Could you check a few things on this model? Use its own coordinates, in mm. A direction names the side the tool comes from. Give positions to 0.01 mm unless a question says otherwise; leave off trailing zeros. Order: outer loops, then holes, each group sorted by start corner. A loop starts at its lowest first (then second) coordinate and runs counter-clockwise, first axis right, second up. Notation, with made-up numbers: M 61,72.25 L 106,72.25 A23 cw 106,107.25 Z; hole C 49,5.25 d3. An arc over 180 degrees is marked long. Return JSON: item names as keys, results as strings. Group by question number.
```python
from build123d import *

# Parameters (mm, degrees)
SKETCH1_W           = 300
SKETCH1_H           = 152
BOSS_EXTRUDE1_DEPTH = 62
CUT_EXTRUDE2_DEPTH  = 342.976607387
SKETCH7_R           = 45
SKETCH7_R_2         = 46.06
SKETCH7_R_3         = 22
CUT_EXTRUDE4_DEPTH  = 339.496676498
CUT_EXTRUDE6_DEPTH  = 339.496676498
CUT_EXTRUDE9_DEPTH  = 339.496676498
SHELL2_DEPTH        = 57
CUT_EXTRUDE10_DEPTH = 55


# Read off the part's stored shape, not the designer's step: Shell2
with BuildPart() as part:
    # Sketch1 → Boss-Extrude1 (new body)
    with BuildSketch(Plane.XY):
        with Locations((150, -76)):
            Rectangle(SKETCH1_W, SKETCH1_H)
    extrude(amount=BOSS_EXTRUDE1_DEPTH)

    # Sketch2 → Cut-Extrude2 (cut, through all)
    with BuildSketch(Plane.XY.offset(62)):
        with BuildLine():
            ThreePointArc((51, -127), (14.937554126, -112.062445807), (0, -75.999999905))
            Line((0, -75.999999905), (0, -152))
            Line((0, -152), (300, -152))
            Line((300, -152), (300, -102))
            Line((300, -102), (260.724181003, -136.984282786))
            ThreePointArc((260.724181003, -136.984282786), (252.157366961, -142.186720854), (242.3, -144))
            ThreePointArc((242.3, -144), (239.848083808, -143.891268673), (237.415416722, -143.565928303))
            Line((237.415416722, -143.565928303), (51, -127))
        make_face()
        with BuildLine():
            ThreePointArc((0, -75.999999905), (14.937554193, -39.937554126), (51, -25))
            Line((51, -25), (166.163471247, -7.695622939))
            ThreePointArc((166.163471247, -7.695622939), (190.26153232, -9.61627718), (210.878909402, -22.238845161))
            Line((210.878909402, -22.238845161), (251.946068796, -20.152501272))
            Line((251.946068796, -20.152501272), (300, -102))
            Line((300, -102), (300, 0))
            Line((300, 0), (0, 0))
            Line((0, 0), (0, -75.999999905))
        make_face()
    extrude(amount=-CUT_EXTRUDE2_DEPTH, mode=Mode.SUBTRACT)

    # Sketch7 → Cut-Extrude4 (cut, through all)
    with BuildSketch(Plane.XY.offset(62)):
        with Locations((51, -76)):
            Circle(SKETCH7_R)
        with Locations((174.2, -59)):
            Circle(SKETCH7_R_2)
        with Locations((242.3, -116.3)):
            Circle(SKETCH7_R_3)
    extrude(amount=-CUT_EXTRUDE4_DEPTH, mode=Mode.SUBTRACT)

    # Sketch6 → Cut-Extrude6 (cut, through all)
    with BuildSketch(Plane.XY.offset(62)):
        with BuildLine():
            Line((95.491028227, -124.62889745), (178.491028227, -132.004746901))
            ThreePointArc((178.491028227, -132.004746901), (184.727429418, -126.786289256), (179.508971773, -120.549888066))
            Line((179.508971773, -120.549888066), (96.508971773, -113.174038615))
            ThreePointArc((96.508971773, -113.174038615), (90.272570582, -118.39249626), (95.491028227, -124.62889745))
        make_face()
    extrude(amount=-CUT_EXTRUDE6_DEPTH, mode=Mode.SUBTRACT)

    # Sketch10 → Cut-Extrude9 (cut, through all)
    with BuildSketch(Plane.XY.offset(62)):
        Polygon((210.878909402, -22.238845161), (223.578909402, -30.744161401), (249.678909402, -30.744161401), (299.082639453, -101.3), (300, -102), (251.946068796, -20.152501272), align=None)
    extrude(amount=-CUT_EXTRUDE9_DEPTH, mode=Mode.SUBTRACT)

    # Shell2 outline → Shell2 (cut)
    with BuildSketch(Plane.XY):
        with BuildLine():
            ThreePointArc((179.951555923, -115.569514659), (189.137709243, -122.70109723), (186.459518175, -134.017995012))
            Line((186.459518175, -134.017995012), (225.572036413, -137.493754604))
            ThreePointArc((225.572036413, -137.493754604), (233.913861687, -90.635380692), (268.314757677, -123.52719745))
            Line((268.314757677, -123.52719745), (293.090088132, -101.458983754))
            Line((293.090088132, -101.458983754), (247.076074149, -35.744161401))
            Line((247.076074149, -35.744161401), (222.05928739, -35.744161401))
            Line((222.05928739, -35.744161401), (218.263483983, -33.202074129))
            ThreePointArc((218.263483983, -33.202074129), (161.890244674, -108.553945593), (147.330636825, -15.581560109))
            Line((147.330636825, -15.581560109), (64.89221906, -27.968695108))
            ThreePointArc((64.89221906, -27.968695108), (100.988642148, -74.934328279), (66.926556679, -123.39561997))
            Line((66.926556679, -123.39561997), (87.292394522, -125.205443511))
            ThreePointArc((87.292394522, -125.205443511), (86.651779504, -113.593617849), (96.951555923, -108.193665208))
            Line((96.951555923, -108.193665208), (179.951555923, -115.569514659))
        make_face()
    extrude(amount=SHELL2_DEPTH, mode=Mode.SUBTRACT)

    # Sketch12 → Cut-Extrude10 (cut)
    with BuildSketch(Plane(origin=(0, 0, 0), x_dir=(-1, 0, 0), z_dir=(0, 0, -1))):
        with BuildLine():
            Line((-64.89221906, -27.968695108), (-51, -31))
            ThreePointArc((-51, -31), (-96, -76), (-51, -121))
            Line((-51, -121), (-66.926556679, -123.39561997))
            ThreePointArc((-66.926556679, -123.39561997), (-100.988642148, -74.934328279), (-64.89221906, -27.968695108))
        make_face()
        with BuildLine():
            Line((-268.314757677, -123.52719745), (-259.127186744, -130.472007137))
            ThreePointArc((-259.127186744, -130.472007137), (-235.806137419, -95.280253361), (-236.398748795, -137.493754604))
            Line((-236.398748795, -137.493754604), (-225.572036413, -137.493754604))
            ThreePointArc((-225.572036413, -137.493754604), (-233.913861687, -90.635380692), (-268.314757677, -123.52719745))
        make_face()
        with BuildLine():
            Line((-186.459518175, -134.017995012), (-87.292394522, -125.205443511))
            ThreePointArc((-87.292394522, -125.205443511), (-86.651779504, -113.593617849), (-96.951555923, -108.193665208))
            Line((-96.951555923, -108.193665208), (-179.951555923, -115.569514659))
            ThreePointArc((-179.951555923, -115.569514659), (-189.137709243, -122.70109723), (-186.459518175, -134.017995012))
        make_face()
        with BuildLine():
            Line((-218.263483983, -33.202074129), (-200.666763454, -21.30339495))
            ThreePointArc((-200.666763454, -21.30339495), (-163.274286328, -103.745417428), (-168.084950709, -13.347729825))
            Line((-168.084950709, -13.347729825), (-147.330636825, -15.581560109))
            ThreePointArc((-147.330636825, -15.581560109), (-161.890244675, -108.553945593), (-218.263483983, -33.202074129))
        make_face()
    extrude(amount=-CUT_EXTRUDE10_DEPTH, mode=Mode.SUBTRACT)


solid = part.part
```
1. Imagine slicing it at B-B, the plane y = -59. Please give me the cut outline in (x, z).
2. If we mould it in two halves opening along X, with no side actions, what happens to faces 6 (the flat face through (274.035, -65.528, 31.434)), 7 (the flat face through (107.78, -16.47, 31.43)), 8 (the flat face through (144, -94, 55))? For each: pulls with the +X half, pulls with the -X half, needs draft (parallel to the pull), parting line crosses it, or undercut.
3. Imagine slicing it at C-C, the plane x = 174.2. Please give me the cut outline in (y, z).
4. Which directions (+Z, -Z, +X, -X, +Y, -Y) give clear straight access to the entire face, cutting with the end or side of a thin tool? Please do faces 1 (the flat face through (138, -131, 0)), 2 (the flat face through (138, -114, 55)), 3 (the flat face through (136.41, -128.265, 58.549)), 4 (the flat face through (280.637, -119.247, 31.434)), 5 (the flat face through (236, -30.744, 31)).
5. Imagine slicing it at D-D, the plane x = 104. Please give me the cut outline in (y, z).
6. I need wall thicknesses on L1, parallel to Y at x = 51, z = 31; L2, parallel to Y at x = 242.3, z = 42; L3, parallel to X at y = -89, z = 53. Which ranges of each line are inside material? Lowest first, please. Write a range as from..to.
7. For pin 1 (10 mm diameter, centred on y = -30.5, z = 32, fed in from +X); pin 2 (24 mm diameter, centred on x = 237.5, y = -102, fed in from -Z); pin 3 (5 mm diameter, centred on y = -115.5, z = 17.5, fed in from +X), each with a flat end and sliding along its axis, tell me the tip position at first contact or that it passes through.
8. Imagine slicing it at A-A, the plane z = 13. Please give me the cut outline in (x, y).
Values:
{
 "1": {"outline": "M 2.92,0 L 9.33,0 L 9.33,62 L 2.92,62 Z; M 92.67,55 L 98.02,55 L 98.02,57 L 123.14,57 L 123.14,55 L 128.14,55 L 128.14,62 L 92.67,62 Z; M 220.26,55 L 225.26,55 L 225.26,57 L 263.36,57 L 263.36,0 L 269.46,0 L 269.46,62 L 220.26,62 Z"},
 "2": {"face 6": "pulls with the +X half", "face 7": "pulls with the -X half", "face 8": "undercut"},
 "3": {"outline": "M -137.95,0 L -132.93,0 L -132.93,55 L -131.62,55 L -131.62,62 L -137.95,62 Z; M -120.08,55 L -115.06,55 L -115.06,57 L -110.06,57 L -110.06,55 L -105.06,55 L -105.06,62 L -120.08,62 Z; M -12.94,0 L -7.07,0 L -7.07,62 L -12.94,62 Z"},
 "4": {"face 1": "-Z, +X, -X, +Y, -Y", "face 2": "-Z", "face 3": "+Z, -Z", "face 4": "+Z, -Z, +X, -Y", "face 5": "+Z, -Z, +X, +Y"},
 "5": {"outline": "M -131.71,0 L -126.69,0 L -126.69,55 L -125.39,55 L -125.39,62 L -131.71,62 Z; M -113.84,55 L -108.82,55 L -108.82,57 L -22.09,57 L -22.09,0 L -17.04,0 L -17.04,62 L -113.84,62 Z"},
 "6": {"L1": "y = -127..-121, -31..-25", "L2": "y = -144..-138.3, -35.74..-30.74", "L3": "x = 1.68..7.92, 284.37..290.47"},
 "7": {"pin 1": "stops at x = 253.01", "pin 2": "stops at z = 55", "pin 3": "stops at x = 287.65"},
 "8": {"outline": "M 51,-127 L 237.42,-143.57 A27.7 ccw 260.72,-136.98 L 300,-102 L 299.08,-101.3 L 249.68,-30.74 L 223.58,-30.74 L 210.88,-22.24 A51.93 ccw 166.16,-7.7 L 51,-25 A51 ccw Z; hole M 51,-121 L 66.93,-123.4 L 225.57,-137.49 L 236.4,-137.49 A22 ccw 259.13,-130.47 L 268.31,-123.53 L 293.09,-101.46 L 247.08,-35.74 L 222.06,-35.74 L 218.26,-33.2 L 200.67,-21.3 A46.06 ccw 168.08,-13.35 L 147.33,-15.58 L 64.89,-27.97 L 51,-31 A45 ccw Z"}
}
